```python
from build123d import *

# Parameters (mm, degrees)
F1_DEPTH = 25.4


with BuildPart() as f1:
    # F0 (on Top) → F1 (new body)
    with BuildSketch(Plane.XY):
        Polygon((-20.0724594905, -35.6141963687), (1.793154165, -15.5119398539), (-14.198616368, -6.4988439839), align=None)
        Polygon((1.793154165, -15.5119398539), (15.306846589, -3.0880620772), (7.6669972876, 13.6034125308), (-10.5683816736, 11.4954333843), (-14.198616368, -6.4988439839), align=None)
        Polygon((-10.5683816736, 11.4954333843), (7.6669972876, 13.6034125308), (-4.694538551, 40.6107857691), align=None)
        Polygon((27.6683824276, -30.0954353155), (15.306846589, -3.0880620772), (1.793154165, -15.5119398539), align=None)
    extrude(amount=F1_DEPTH)


solid = f1.part
```
Geometry check sheet. Reference: the model listing, model coordinates, mm. A direction names the side the tool comes from. Give positions to 0.01 mm unless a question says otherwise; leave off trailing zeros. Write each loop counter-clockwise with the first axis right and the second up, starting at its lowest first coordinate (ties: lowest second). Pieces come first, ordered by that corner, then holes. Notation, with made-up numbers: (-15.5, 15) -> (19.5, 15) arc R30 ccw to (19.5, 48) -> close; hole circle Ø10 at (77, 69). An arc over 180 degrees is marked (long way). Use one line per item in the form item = value.
Item 1: Sectioned sample at A-A on y = -29. Enter the section's corners in (x, z).
Results list:
outline = (-18.74, 0) -> (-12.88, 0) -> (-12.88, 25.4) -> (-18.74, 25.4) -> close; (25.72, 0) -> (27.17, 0) -> (27.17, 25.4) -> (25.72, 25.4) -> close
Item 2: Sectioned sample at D-D on x = 8.5. Enter the section's corners in (y, z).
Results list:
outline = (-19.29, 0) -> (11.78, 0) -> (11.78, 25.4) -> (-19.29, 25.4) -> close
Item 3: Sectioned sample at B-B on z = 14. Enter the section's corners in (x, y).
Results list:
outline = (-20.07, -35.61) -> (1.79, -15.51) -> (27.67, -30.1) -> (-4.69, 40.61) -> close
Item 4: Scan lines: line 1 (X direction, y = -17, z = 11); line 2 (X direction, y = -19.5, z = 6.25); line 3 (X direction, y = 3, z = 13.5). Record each from-to range of solid material in increasing order.
Results list:
line_1 = -16.32 to 0.17, 4.43 to 21.67
line_2 = -16.82 to -2.54, 8.87 to 22.82
line_3 = -12.28 to 12.52
Item 5: Depth check by flat-ended pin: pin 1 Ø12 at (x, z) = (-7, 3.5) entering from -Y; pin 2 Ø1 at (y, z) = (20.5, 21.5) entering from -X; pin 3 Ø8 at (y, z) = (-13.5, 19) entering from -X. Enter the tip coordinate at first touch or a pass-through.
Results list:
pin_1 = -29.11
pin_2 = -8.85
pin_3 = -16.42
Item 6: Mould release check, pull along X, two halves, no side actions. Record for faces 3 (the flat face through (14.55, -22.7, 12.52)), 4 (the flat face through (-2, -5, 0)): released by +X, released by -X, zero draft, split by the parting line, or undercut.
Results list:
face_3 = undercut
face_4 = zero draft
Item 7: Sectioned sample at C-C on y = 12.5. Enter the section's corners in (x, z), plus the area to 3 significant figures.
Results list:
outline = (-10.37, 0) -> (8.17, 0) -> (8.17, 25.4) -> (-10.37, 25.4) -> close
area = 471 mm2
Item 8: Access from +Z, -Z, +X, -X, +Y, -Y to the whole of each face (thin tool, end or side, straight path). Record for faces 1 (the flat face through (-9.29, -25.7, 12.52)), 2 (the flat face through (-2, -5, 25.4)).
Results list:
face_1 = +Z, -Z, -Y
face_2 = +Z, +X, -X, +Y, -Y
